Autodesk Inventor part; units mm, degrees
ref_plane "YZ Plane" through (0, 0, 0) normal (1, 0, 0) x (0, 1, 0)
ref_plane "XZ Plane" through (0, 0, 0) normal (0, 1, 0) x (-1, 0, 0)
ref_plane "XY Plane" through (0, 0, 0) normal (0, 0, 1) x (1, 0, 0)
sketch "Sketch1" plane through (0, 0, 0) normal (0, 1, 0) x (-1, 0, 0)
  line L0 (0, 0) -> (38.1, 0)
  line L1 (38.1, 0) -> (38.1, -38.1)
  line L2 (38.1, -38.1) -> (0, -38.1)
  line L3 (0, -38.1) -> (0, 0)
  line L4 (0, -38.1) -> (0, -31.75)
  line L5 (0, -38.1) -> (6.35, -38.1) construction
  line L6 (0, -31.75) -> (25.4, -31.75)
  line L7 (25.4, -31.75) -> (25.4, -6.35)
  line L8 (0, 0) -> (0, -38.1)
  line L9 (0, 0) -> (38.1, 0)
  line L10 (38.1, 0) -> (38.1, 12.7)
  line L11 (38.1, 12.7) -> (0, 12.7)
  line L12 (0, 12.7) -> (0, 0)
  dimension "d0" = 38.1
  dimension "d1" = 38.1
  dimension "d2" = 6.35
  dimension "d3" = 90
  dimension "d4" = 25.4
  dimension "d5" = 90
  dimension "d6" = 25.4
  dimension "d34" = 38.1
  dimension "d35" = 12.7
extrude "Extrusion1" add sketch "Sketch1" along normal blind 56.896
hole "Hole1" at (-25.4, 0, -31.75) at (-25.4, 0, -6.35) direction (0, 1, 0) diameter 9.2075 depth 12.7
sketch "Sketch2" plane through (-38.1, 0, -38.1) normal (-1, 0, 0) x (0, 0, 1)
  line L0 (19.05, 0) -> (19.05, 17.78)
  line L1 (19.05, 0) -> (36.83, 0) construction
  line L2 (19.05, 17.78) -> (19.05, 27.686)
  line L3 (19.05, 17.78) -> (28.956, 17.78) construction
  line L4 (19.05, 27.686) -> (19.05, 32.766)
  line L5 (19.05, 32.766) -> (19.05, 42.672)
  circle A0 centre (19.05, 17.78) radius 9.906
  circle A1 centre (19.05, 42.672) radius 9.906
  ellipse E0 centre (19.05, 42.672) end of major axis (28.702, 42.672) minor radius 3.5267
  ellipse E1 centre (19.05, 17.78) end of major axis (28.956, 17.78) minor radius 3.6751
  line L6 (19.05, 42.672) -> (19.05, 57.404)
  line L7 (19.05, 30.226) -> (29.21, 30.226)
  line L8 (29.21, 30.226) -> (39.116, 30.226)
  circle A2 centre (39.116, 30.226) radius 9.906
  ellipse E2 centre (39.116, 30.226) end of major axis (29.21, 30.226) minor radius 3.1895
  dimension "d16" = 17.78
  dimension "d17" = 90
  dimension "d18" = 9.906
  dimension "d19" = 90
  dimension "d20" = 5.08
  dimension "d21" = 180
  dimension "d22" = 9.906
  dimension "d23" = 180
  dimension "d32" = 14.732
  dimension "d36" = 10.16
  dimension "d37" = 9.906
  dimension "d38" = 19.812
extrude "Extrusion2" cut sketch "Sketch2" against normal blind 31.75
extrude "Extrusion3" cut sketch "Sketch2" against normal blind 38.1 contours E2 | E1 L2 L0 | L0 L2 E1 | E0 L6 L5 | L5 L6 E0
sketch "Sketch3" plane through (0, 0, 0) normal (1, 0, 0) x (0, 0, -1)
  line L0 (38.1, 0) -> (38.1, 56.896)
  line L1 (0, 44.577) -> (38.1, 44.577)
  line L2 (38.1, 44.577) -> (38.1, 40.767)
  line L3 (38.1, 40.767) -> (0, 40.767)
  line L4 (0, 40.767) -> (0, 44.577)
  line L5 (0, 44.577) -> (38.1, 40.767) construction
  line L6 (38.1, 44.577) -> (0, 40.767) construction
  line L7 (0, 19.685) -> (38.1, 19.685)
  line L8 (38.1, 19.685) -> (38.1, 15.875)
  line L9 (38.1, 15.875) -> (0, 15.875)
  line L10 (0, 15.875) -> (0, 19.685)
  line L11 (0, 19.685) -> (38.1, 15.875) construction
  line L12 (38.1, 19.685) -> (0, 15.875) construction
  line L13 (-12.7, 0) -> (-12.7, 56.896)
  line L14 (0, 15.875) -> (-12.7, 15.875)
  line L15 (-12.7, 15.875) -> (-12.7, 19.685)
  line L16 (-12.7, 19.685) -> (0, 19.685)
  line L17 (0, 19.685) -> (0, 15.875)
  line L18 (0, 40.767) -> (-12.7, 40.767)
  line L19 (-12.7, 40.767) -> (-12.7, 44.577)
  line L20 (-12.7, 44.577) -> (0, 44.577)
  line L21 (0, 44.577) -> (0, 40.767)
  line L22 (-12.7, 0) -> (-12.7, 56.896)
  line L23 (38.1, 0) -> (38.1, 56.896)
  line L24 (-40.132, 28.321) -> (38.1, 28.321)
  line L25 (38.1, 28.321) -> (38.1, 32.131)
  line L26 (38.1, 32.131) -> (-40.132, 32.131)
  line L27 (-40.132, 32.131) -> (-40.132, 28.321)
  line L28 (-40.132, 28.321) -> (38.1, 32.131) construction
  line L29 (38.1, 28.321) -> (-40.132, 32.131) construction
  point P0 (0, 0)
  point P1 (19.05, 17.78)
  point P2 (19.05, 42.672)
  point P3 (-1.016, 30.226)
  point P4 (38.1, 28.321)
  dimension "d28" = 3.81
  dimension "d29" = 3.81
  dimension "d39" = 3.81
extrude "Extrusion4" cut sketch "Sketch3" against normal blind 6.35 contours L9 L10 L7 L0 | L14 L13 L16 L10 | L24 L13 L26 L0 | L24 L27 L26 L13 | L3 L4 L1 L0 | L18 L13 L20 L4
fillet "Fillet1" radius 3.175 2 edges at (-38.1, 56.896, -12.7) (-38.1, 28.448, 12.7)
properties part number "Valve Holder-3valve"
Verification items for the finished model (mm, model axes). A direction names the side the tool comes from. Coordinates: 2 decimals unless noted, no trailing zeros. Write each loop counter-clockwise with the first axis right and the second up, starting at its lowest first coordinate (ties: lowest second). Pieces come first, ordered by that corner, then holes. Notation, with made-up numbers: (24.25, 60.5) -> (32.25, 60.5) arc R19 cw to (32.25, 91.5) -> close; hole circle Ø9 at (33, -15.5). An arc over 180 degrees is marked (long way). One line per item, written item: value. Start each with the question number.
Q1. Cross-section at D-D on y = 51. Enter the section's corners in (x, z) (3 decimals).
Q2. Cross-section at C-C on z = -31.75. Enter the section's corners in (x, y) (3 decimals).
Q3. Go/stop test with flat-tipped pins: P1, Ø10, axis at y = 25.5, z = 6.5, coming from the +X side; P2, Ø5.5, axis at x = -25.4, z = -6.35, coming from the -Y side; P3, Ø16, axis at y = 17.78, z = -19.05, coming from the -X side; P4, Ø3, axis at y = 42.5, z = 3.5, coming from the +X side. Record where each tip stops, or that it passes through.
Q4. Access from +Z, -Z, +X, -X, +Y, -Y to the whole of each face (thin tool, end or side, straight path). Record for faces 1 (the cylindrical face through (-37.19, 46.25, 11.75)), 2 (the flat face through (-6.35, 49, -19)), 3 (the flat face through (-3, 44.577, 1)), 4 (the flat face through (-25, 12.7, -32)).
Q5. Mould release check, pull along Z, two halves, no side actions. Record for faces 5 (the flat face through (-17, 56.896, -12)), 6 (the flat face through (-18, 28, 12.7)), 7 (the flat face through (-6.35, 24, -19)), 8 (the flat face through (-6.35, 36, 1)): pulls with the +Z half, pulls with the -Z half, needs draft (parallel to the pull), parting line crosses it, or undercut.
Q6. Cross-section at B-B on x = -29. Enter the section's corners in (y, z).
Q7. Cross-section at A-A on y = 41.5. Enter the section's corners in (x, z) (3 decimals), and give its area (3 significant figures).
Q8. Thickness scan on L1, parallel to Z at x = -25.4, y = 6.5; L2, parallel to Y at x = -14, z = -19; L3, parallel to Y at x = -3, z = -10.5 (3 decimals). Record the ranges inside material, lowest first. Write a range as from..to.
Checked values:
1. outline: (-38.1, -38.1) -> (0, -38.1) -> (0, 12.7) -> (-34.925, 12.7) arc R3.175 ccw to (-38.1, 9.525) -> (-38.1, -13.686) -> (-6.35, -13.686) -> (-6.35, -24.414) -> (-38.1, -24.414) -> close
2. outline: (-38.1, 0) -> (-30.004, 0) -> (-30.004, 12.7) -> (-20.796, 12.7) -> (-20.796, 0) -> (0, 0) -> (0, 15.875) -> (-6.35, 15.875) -> (-6.35, 19.685) -> (0, 19.685) -> (0, 28.321) -> (-6.35, 28.321) -> (-6.35, 32.131) -> (0, 32.131) -> (0, 40.767) -> (-6.35, 40.767) -> (-6.35, 44.577) -> (0, 44.577) -> (0, 56.896) -> (-34.925, 56.896) arc R3.175 ccw to (-38.1, 53.721) -> close
3. P1: stops at x = 0
3. P2: stops at y = 12.7
3. P3: stops at x = -6.35
3. P4: stops at x = -6.35
4. face 1: +Z, -X, +Y
4. face 2: -X
4. face 3: +Z, -Z, +X
4. face 4: -Y
5. face 5: needs draft
5. face 6: pulls with the +Z half
5. face 7: undercut
5. face 8: undercut
6. outline: (0, -38.1) -> (56.9, -38.1) -> (56.9, 12.7) -> (0, 12.7) -> (0, -3.48) -> (12.7, -3.48) -> (12.7, -9.22) -> (0, -9.22) -> (0, -28.88) -> (12.7, -28.88) -> (12.7, -34.62) -> (0, -34.62) -> close; hole circle Ø19.81 at (17.78, -19.05); hole circle Ø19.81 at (30.23, 1.02); hole circle Ø19.81 at (42.67, -19.05)
7. outline: (-38.1, -38.1) -> (-6.35, -38.1) -> (-6.35, -28.886) -> (-38.1, -28.886) -> close; (-38.1, -9.214) -> (-6.35, -9.214) -> (-6.35, 12.7) -> (-34.925, 12.7) arc R3.175 ccw to (-38.1, 9.525) -> close
7. area: 986 mm²
8. L1: z = -38.1..-36.35, -27.15..-10.95, -1.75..12.7
8. L2: y = 0..7.87, 27.69..32.77, 52.58..56.9
8. L3: y = 0..15.875, 19.685..28.321, 32.131..40.767, 44.577..56.896
